Could you check a few things on this model? Use its own coordinates, in mm. A direction names the side the tool comes from. Give positions to 0.01 mm unless a question says otherwise; leave off trailing zeros. Loops run counter-clockwise (first coordinate to the right, second up) from the corner with the lowest first, then second, coordinate; pieces in that order, holes last.
1. Imagine slicing it at B-B (x = -3). List the corners of the cut face in (y, z) for me.
2. Thinking about a two-plate mould opening in X: for faces 3 (the cylindrical face through (0.07, 0.08, 1.14)), 4 (the cylindrical face through (2.7, 13.4, 1.2)), 5 (the cylindrical face through (-2.676, 0.006, -13.468)), which applies, +X half, -X half, draft (parallel to the pull), parting line (faces both ways), or undercut?
3. Imagine slicing it at A-A (z = -11). List the corners of the cut face in (x, y) for me, plus the area to 3 significant figures.
4. Imagine slicing it at C-C (y = 3). List the corners of the cut face in (x, z) for me, plus the area to 3 significant figures.
5. For P1, Ø6, axis at x = 1.5, z = -3, coming from the +Y side, with a flat end and sliding along its axis, tell me the tip position at first contact or that it passes through.
6. Imagine slicing it at D-D (x = 1). Count the separate pieces of the cut face and the enclosed holes in it, plus the area to 3 significant figures.
7. For faces 1 (the flat face through (2.3, 0.4, -6.9)), 2 (the flat face through (5, 0, -2)), which set-ups out of +Z, -Z, +X, -X, +Y, -Y let a thin tool reach every point of the face, with its end or its side?
8. I need wall thicknesses on line 1 along Z through (x, y) = (-3.5, 5); line 2 along Y through (x, z) = (-1.5, -13); line 3 along Y through (x, z) = (-0.75, 1.25). Which ranges of each line are inside material? Lowest first, please.
Autodesk Inventor part; units mm, degrees
ref_plane "YZ Plane" through (0, 0, 0) normal (1, 0, 0) x (0, 1, 0)
ref_plane "XZ Plane" through (0, 0, 0) normal (0, 1, 0) x (-1, 0, 0)
ref_plane "XY Plane" through (0, 0, 0) normal (0, 0, 1) x (1, 0, 0)
sketch "Эскиз1" plane through (0, 0, 0) normal (0, 1, 0) x (-1, 0, 0)
  line L0 (5, -14) -> (-5, -14)
  line L1 (-5, -14) -> (-5, 0)
  line L2 (-5, 0) -> (5, 0)
  line L3 (5, 0) -> (5, -14)
  line L4 (0, -10.25) -> (0, -3.75)
  line L5 (0, -14) -> (0, 0) construction
  ellipse E0 centre (0, -7) end of major axis (-2.075, -7) minor radius 3.25
  dimension "d5" = 2.075
  dimension "d0" = 14
  dimension "d1" = 10
  dimension "d4" = 6.5
extrude "Выдавливание1" add sketch "Эскиз1" along normal mid plane 0.8
mirror "Зеркальное отражение1" about plane through (0, 0, 0) normal (0, 0, 1) of "Выдавливание1"
sketch "Эскиз2" plane through (0, 0.4, 0) normal (0, 1, 0) x (1, 0, 0)
  point P0 (0, 0)
sketch "Эскиз3" plane through (0, 0.4, 0) normal (0, 1, 0) x (1, 0, 0)
  ellipse E0 centre (0, 7) end of major axis (0, 10.25) minor radius 2.075
  line L0 (5, 14) -> (-5, 14)
  arc A0 (5, 11.899) -> (0, 14) centre (0, 7) ccw
  arc A1 (0, 14) -> (-5, 11.899) centre (0, 7) ccw
  line L1 (5, 14) -> (5, -14)
  line L2 (-5, 14) -> (-5, -14)
  line L3 (2.799, 0) -> (-2.799, 0) construction
  arc A2 (0, -14) -> (5, -11.899) centre (0, -7) ccw
  arc A3 (-5, -11.899) -> (0, -14) centre (0, -7) ccw
  line L4 (5, -14) -> (-5, -14)
  point P0 (0, 0)
  point P1 (0, 0)
  point P2 (5, -11.899)
extrude "Выдавливание2" cut sketch "Эскиз3" against normal up to surface (0.8 mm away) contours L1 A0 L0 | A1 L2 L0 | L1 L4 A2 | A3 L4 L2
sketch "Эскиз5" plane through (0, 0.4, 0) normal (0, 1, 0) x (1, 0, 0)
  line L0 (-5, 11.899) -> (-5, -11.899)
  line L1 (-5, 0) -> (5, 0)
  line L2 (5, 11.899) -> (5, -11.899)
  point P0 (0, 0)
bend part "Сгиб детали1" radius 0.8 angle 90 line through (-5, 0.4, 0) along (1, 0, 0) centre toward (0, 1, 0) moving side (0, 0, 1) both sides no
equation "\"Радиус_гибки\" = Толщина"
equation "\"Ширина_просечки\" = Толщина"
equation "\"Глубина_просечки\" = 0.5 * Толщина"
equation "\"Размер_просечки\" = 4 * Толщина"
equation "\"Мин_остаток\" = 2 * Толщина"
equation "\"Радиус_перехода\" = Радиус_гибки"
equation "\"Радиус_Якоби\" = Радиус_гибки"
equation "\"Размер_зазора\" = Толщина"
properties part number "Уголок"
Derived:
1. outline: (-0.4, -13.32) - (0.4, -13.32) - (0.4, 0) arc R0.8 cw to (1.2, 0.8) - (13.27, 0.8) - (13.27, 1.6) - (1.2, 1.6) arc R1.6 ccw to (-0.4, 0) - close
2. face 3: draft
2. face 4: +X half
2. face 5: -X half
3. outline: (-5, -0.4) - (5, -0.4) - (5, 0.4) - (-5, 0.4) - close
3. area: 8.00 mm2
4. outline: (-5, 0.8) - (5, 0.8) - (5, 1.6) - (-5, 1.6) - close
4. area: 8.00 mm2
5. P1: stops at y = 0.4
6. separate pieces: 3
6. enclosed holes: 0
6. area: 13.7 mm2
7. face 1: -Z, +X, -X, +Y
7. face 2: +Z, -Z, +X, +Y, -Y
8. line 1: z = 0.8 to 1.6
8. line 2: y = -0.4 to 0.4
8. line 3: y = 0.2 to 3.91, 9.97 to 13.9
